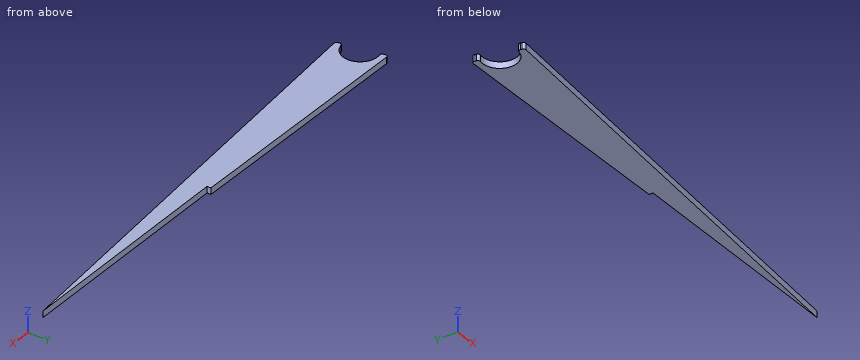
```python
from build123d import *

# Parameters (mm, degrees)
SM_BASE_FLANGE_1_DEPTH = 5


# Sheet-metal steps are written as plain solids
with BuildPart() as part:
    # Sketch 1 → Базовая кромка1 (new body)
    with BuildSketch(Plane.XY):
        with BuildLine():
            Line((1.279191503, -33.168907268), (1.064618958, -32.092874536))
            ThreePointArc((1.064618958, -32.092874536), (1.362719913, -30.59112672), (2.635550334, -29.740236948))
            ThreePointArc((2.635550334, -29.740236948), (13.239337122, -13.859933227), (-2.644582905, -3.261564244))
            ThreePointArc((-2.644582905, -3.261564244), (-4.146432324, -2.963975592), (-4.997756242, -1.691435506))
            Line((-4.997756242, -1.691435506), (-5.212328788, -0.615402774))
            ThreePointArc((-5.212328788, -0.615402774), (-4.791260853, 1.051425345), (-3.232048448, 1.775628952))
            Line((-3.232048448, 1.775628952), (184.68601887, 0))
            Line((184.68601887, 0), (184.68601887, -3))
            Line((184.68601887, -3), (362.597814819, -3))
            Line((362.597814819, -3), (3.416789292, -34.770008252))
            ThreePointArc((3.416789292, -34.770008252), (2.041580213, -34.378539846), (1.279191503, -33.168907268))
        make_face()
    extrude(amount=-SM_BASE_FLANGE_1_DEPTH)


solid = part.part
```
Input: part model. Units: mm. Frame: model coordinates. Round coordinates to 2 decimals unless told otherwise and drop trailing zeros. Loops run counter-clockwise (first coordinate to the right, second up) from the corner with the lowest first, then second, coordinate; pieces in that order, holes last. Notation, with made-up numbers: (31.5, 87) -> (76.5, 87) arc R11 ccw to (76.5, 105) -> close; hole circle Ø4 at (-22, 41). An arc over 180 degrees is marked (long way). One line per item, written item: value.
(1) Section C-C (y = -14). Return the cut outline in (x, z), plus the area to 3 significant figures.
Geometry check:
outline: (13.27, -5) -> (238.24, -5) -> (238.24, 0) -> (13.27, 0) -> close
area: 1,120 mm2
(2) Section B-B (x = 32). Return the cut outline in (y, z), plus the area to 3 significant figures.
Geometry check:
outline: (-32.24, -5) -> (1.44, -5) -> (1.44, 0) -> (-32.24, 0) -> close
area: 168 mm2
(3) Material intervals for line 1 (X direction, y = -0.5, z = -2.85); line 2 (Y direction, x = 30, z = -4.45); line 3 (Y direction, x = 145, z = -2.7) (3 decimals), sorted ascending. Write a range as [from, to].
Geometry check:
line 1: [-5.23, 184.69]
line 2: [-32.42, 1.46]
line 3: [-22.247, 0.375]
(4) Section A-A (z = -2.95). Return the cut outline in (x, y), plus the area to 3 significant figures.
Geometry check:
outline: (-5.21, -0.62) -> (-5, -1.69) arc R2 ccw to (-2.64, -3.26) arc R13.5 cw to (2.64, -29.74) arc R2 ccw to (1.06, -32.09) -> (1.28, -33.17) arc R2 ccw to (3.42, -34.77) -> (362.6, -3) -> (184.69, -3) -> (184.69, 0) -> (-3.23, 1.78) arc R2 ccw to start
area: 6,260 mm2
(5) Pin query (flat end, axial travel): pin 1 (0.9 mm diameter, centred on y = -2, z = -2.5, fed in from +X); pin 2 (1 mm diameter, centred on x = 60, z = -1, fed in from +Y); pin 3 (2 mm diameter, centred on y = -9.5, z = -4, fed in from -X). Return the tip coordinate at first contact, or that it passes through.
Geometry check:
pin 1: x = 184.69
pin 2: y = 1.18
pin 3: x = 10.87
